Here's how the part is built. I have some questions about the finished solid (model axes, mm). Face numbers are marked on the shaded views. A direction names the side the tool comes from. Coordinates: 2 decimals unless noted, no trailing zeros. Order: outer loops, then holes, each group sorted by start corner. A loop starts at its lowest first (then second) coordinate and runs counter-clockwise, first axis right, second up. Notation, with made-up numbers: (-28.75, 24) -> (8.25, 24) arc R16 ccw to (8.25, 53) -> close; hole circle Ø5 at (81.25, 15). An arc over 180 degrees is marked (long way). One line per item, written item: value. Start each with the question number.
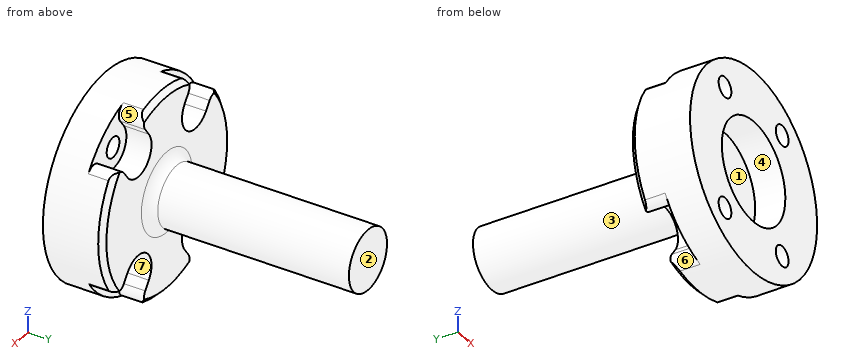
```python
from build123d import *

# Parameters (mm, degrees)
SKETCH_2_R          = 1.0000000000000002
SKETCH_2_R_2        = 0.9999999999999998
CUT_EXTRUDE_1_DEPTH = 10
SKETCH_3_R          = 1.0000000000000002
SKETCH_3_R_2        = 0.9999999999999998
CUT_EXTRUDE_2_DEPTH = 2.5
FILLET_1_R          = 1
FILLET_2_R          = 1


with BuildPart() as part:
    # 草图1 → 旋转1 (revolve)
    with BuildSketch(Plane.XY, mode=Mode.PRIVATE) as revolve_1_sk:
        Polygon((-1.97e-15, 26), (2.999999999999997, 26), (3, 6), (9.5, 5.999999999999999), (10.000000000000002, 5.5), (10, -1.2e-16), (5.000000000000001, -6.1e-16), (5.000000000000002, 2.9999999999999996), (8.7e-16, 2.999999999999999), align=None)
    revolve(revolve_1_sk.sketch.rotate(Axis((0, 9.947317903416637, 0), (0, -1, 0)), 90), axis=Axis((0, 9.947317903416637, 0), (0, -1, 0)))

    # 草图2 → 切除-拉伸1 (cut)
    with BuildSketch(Plane(origin=(0, 6, 0), x_dir=(1, 0, 0), z_dir=(0, 1, 0))):
        with Locations(Location((-4.5, 6.000000000000001, 0), (0, 0, 270))):
            Circle(SKETCH_2_R)
        with Locations(Location((4.5, 6.000000000000003, 0), (0, 0, 270))):
            Circle(SKETCH_2_R_2)
        with Locations(Location((4.5, -5.999999999999997, 0), (0, 0, 270))):
            Circle(SKETCH_2_R_2)
        with Locations(Location((-4.5, -5.999999999999999, 0), (0, 0, 270))):
            Circle(SKETCH_2_R)
    extrude(amount=-CUT_EXTRUDE_1_DEPTH, mode=Mode.SUBTRACT)

    # 草图3 → 切除-拉伸2 (cut)
    # profile 1 of 8: a face of its own
    with BuildSketch(Plane(origin=(0, 6, 0), x_dir=(1, 0, 0), z_dir=(0, 1, 0))):
        with BuildLine():
            Line((-9.157565431651806, 8.710087242202405), (-7.2389927145122455, 6.151990286016327))
            ThreePointArc((-7.2389927145121735, 6.151990286016362), (-5.700000000000015, 7.599999999999989), (-3.8789927145123357, 8.67199028601625))
            Line((-3.8789927145122554, 8.67199028601634), (-5.797565431651803, 11.230087242202407))
            Line((-5.797565431651803, 11.230087242202407), (-9.157565431651806, 8.710087242202405))
        make_face()
    # profile 2 of 8: a face of its own
    with BuildSketch(Plane(origin=(0, 6, 0), x_dir=(1, 0, 0), z_dir=(0, 1, 0))):
        with BuildLine():
            ThreePointArc((-3.8789927145123357, 8.67199028601625), (-5.700000000000015, 7.599999999999989), (-7.2389927145121735, 6.151990286016362))
            Line((-7.2389927145122455, 6.151990286016327), (-6.18, 4.739999999999999))
            ThreePointArc((-6.18, 4.739999999999998), (-3.24, 4.3199999999999985), (-2.819999999999999, 7.259999999999998))
            Line((-2.819999999999999, 7.259999999999998), (-3.8789927145122554, 8.67199028601634))
        make_face()
        with Locations(Location((-4.5, 6.000000000000001, 0), (0, 0, 270))):
            Circle(SKETCH_3_R, mode=Mode.SUBTRACT)
    # profile 3 of 8: a face of its own
    with BuildSketch(Plane(origin=(0, 6, 0), x_dir=(1, 0, 0), z_dir=(0, 1, 0))):
        with BuildLine():
            ThreePointArc((7.2389927145121815, 6.1519902860163524), (5.700000000000022, 7.599999999999984), (3.878992714512337, 8.67199028601625))
            Line((3.8789927145122567, 8.671990286016342), (2.819999999999999, 7.259999999999998))
            ThreePointArc((2.8199999999999985, 7.259999999999998), (3.24, 4.319999999999999), (6.18, 4.739999999999999))
            Line((6.18, 4.739999999999999), (7.238992714512243, 6.151990286016323))
        make_face()
        with Locations(Location((4.5, 6.000000000000003, 0), (0, 0, 270))):
            Circle(SKETCH_3_R_2, mode=Mode.SUBTRACT)
    # profile 4 of 8: a face of its own
    with BuildSketch(Plane(origin=(0, 6, 0), x_dir=(1, 0, 0), z_dir=(0, 1, 0))):
        with BuildLine():
            Line((5.797565431651803, 11.230087242202407), (3.8789927145122567, 8.671990286016342))
            ThreePointArc((3.878992714512337, 8.67199028601625), (5.700000000000022, 7.599999999999984), (7.2389927145121815, 6.1519902860163524))
            Line((7.238992714512243, 6.151990286016323), (9.157565431651806, 8.710087242202405))
            Line((9.157565431651806, 8.710087242202405), (5.797565431651803, 11.230087242202407))
        make_face()
    # profile 5 of 8: a face of its own
    with BuildSketch(Plane(origin=(0, 6, 0), x_dir=(1, 0, 0), z_dir=(0, 1, 0))):
        with BuildLine():
            Line((2.819999999999999, -7.259999999999998), (3.8789927145122527, -8.671990286016337))
            ThreePointArc((3.8789927145123175, -8.671990286016259), (5.700000000000012, -7.599999999999992), (7.238992714512178, -6.151990286016356))
            Line((7.238992714512243, -6.151990286016323), (6.18, -4.739999999999999))
            ThreePointArc((6.18, -4.739999999999999), (3.24, -4.319999999999999), (2.8199999999999985, -7.259999999999998))
        make_face()
        with Locations(Location((4.5, -5.999999999999997, 0), (0, 0, 270))):
            Circle(SKETCH_3_R_2, mode=Mode.SUBTRACT)
    # profile 6 of 8: a face of its own
    with BuildSketch(Plane(origin=(0, 6, 0), x_dir=(1, 0, 0), z_dir=(0, 1, 0))):
        with BuildLine():
            ThreePointArc((7.238992714512178, -6.151990286016356), (5.700000000000012, -7.599999999999992), (3.8789927145123175, -8.671990286016259))
            Line((3.8789927145122527, -8.671990286016337), (5.797565431651803, -11.230087242202407))
            Line((5.797565431651803, -11.230087242202407), (9.157565431651806, -8.710087242202405))
            Line((9.157565431651806, -8.710087242202405), (7.238992714512243, -6.151990286016323))
        make_face()
    # profile 7 of 8: a face of its own
    with BuildSketch(Plane(origin=(0, 6, 0), x_dir=(1, 0, 0), z_dir=(0, 1, 0))):
        with BuildLine():
            ThreePointArc((-2.819999999999999, -7.259999999999998), (-2.4211060633115498, -5.703015151901651), (-3.239999999999995, -4.320000000000003))
            ThreePointArc((-3.239999999999995, -4.320000000000003), (-4.796984848098346, -3.921106063311549), (-6.18, -4.739999999999998))
            Line((-6.18, -4.739999999999999), (-7.238992714512246, -6.151990286016328))
            ThreePointArc((-7.238992714512174, -6.15199028601636), (-5.7000000000000135, -7.59999999999999), (-3.8789927145123286, -8.671990286016255))
            Line((-3.8789927145122527, -8.671990286016337), (-2.819999999999999, -7.259999999999998))
        make_face()
        with BuildLine():
            ThreePointArc((-3.5, -5.999999999999999), (-5.3944271909999175, -6.447213595499955), (-3.899999999999996, -5.200000000000002))
            ThreePointArc((-3.899999999999996, -5.200000000000002), (-3.605572809000083, -5.5527864045000435), (-3.5, -5.999999999999999))
        make_face(mode=Mode.SUBTRACT)
    # profile 8 of 8: a face of its own
    with BuildSketch(Plane(origin=(0, 6, 0), x_dir=(1, 0, 0), z_dir=(0, 1, 0))):
        with BuildLine():
            ThreePointArc((-3.8789927145123286, -8.671990286016255), (-5.7000000000000135, -7.59999999999999), (-7.238992714512174, -6.15199028601636))
            Line((-7.238992714512246, -6.151990286016328), (-9.157565431651806, -8.710087242202405))
            Line((-9.157565431651806, -8.710087242202405), (-5.797565431651803, -11.230087242202407))
            Line((-5.797565431651803, -11.230087242202407), (-3.8789927145122527, -8.671990286016337))
        make_face()
    extrude(amount=-CUT_EXTRUDE_2_DEPTH, mode=Mode.SUBTRACT)

    # 圆角1
    fillet_1_edges = [part.edges().sort_by_distance(p)[0] for p in [
        (7.5462083154282915, 4.5, -6.56161108723772),
        (4.18620831542829, 4.5, -9.08161108723772),
        (4.18620831542829, 4.5, 9.08161108723772),
        (7.5462083154282915, 4.5, 6.561611087237719),
        (-4.18620831542829, 4.5, 9.08161108723772),
        (-7.546208315428291, 4.5, 6.56161108723772),
        (-7.54620831542829, 4.5, -6.561611087237719),
        (-4.186208315428289, 4.5, -9.08161108723772),
    ]]
    fillet(fillet_1_edges, radius=FILLET_1_R)

    # 圆角2
    fillet_2_edges = [part.edges().sort_by_distance(p)[0] for p in [
        (-7e-16, 6, -3),
    ]]
    fillet(fillet_2_edges, radius=FILLET_2_R)


solid = part.part
```
Q1. Imagine slicing it at B-B (x = 4.5). Write out the boundary of the cut face in (y, z).
Q2. Imagine slicing it at A-A (z = -6.5). Write out the boundary of the cut face in (x, y), plus the area to 3 significant figures.
Q3. Imagine slicing it at D-D (x = 0). Write out the boundary of the cut face in (y, z).
Q4. For P1, Ø5, axis at x = 6.5, z = -5.5, coming from the +Y side; P2, Ø4, axis at x = -2, y = 7, coming from the +Z side; P3, Ø6, axis at x = -3.5, y = 12.5, coming from the -Z side, each with a flat end and sliding along its axis, tell me the tip position at first contact or that it passes through.
Q5. I need wall thicknesses on line 1 (X direction, y = 2.1, z = 0); line 2 (X direction, y = 2.25, z = 6); line 3 (Y direction, x = 7.5, z = -3.5). Which ranges of each line are inside material? Lowest first, please.
Q6. Imagine slicing it at C-C (z = 0). Write out the boundary of the cut face in (x, y), plus the area to 3 significant figures.
Q7. For the marked faces 4, 5, 6 and 7, which set-ups out of +Z, -Z, +X, -X, +Y, -Y let a thin tool reach every point of the face, with its end or its side?
Q8. If we mould it in two halves opening along Z, with no side actions, what happens to the marked faces 1, 2 and 3? For each: +Z half, -Z half, draft (parallel to the pull), parting line (faces both ways), or undercut.
Completed:
1. outline: (0, -8.93) -> (3.5, -8.93) -> (3.5, -7) -> (0, -7) -> close; (0, -5) -> (3.5, -5) -> (3.5, -3.9) -> (6, -3.9) -> (6, 3.9) -> (3.5, 3.9) -> (3.5, 5) -> (0, 5) -> (0, 2.18) -> (3, 2.18) -> (3, -2.18) -> (0, -2.18) -> close; (0, 7) -> (3.5, 7) -> (3.5, 8.93) -> (0, 8.93) -> close
2. outline: (-7.6, 0) -> (-5.37, 0) -> (-5.37, 3.5) -> (-7.6, 3.5) -> close; (-3.63, 0) -> (3.63, 0) -> (3.63, 3.5) -> (2.46, 3.5) -> (2.46, 6) -> (-2.46, 6) -> (-2.46, 3.5) -> (-3.63, 3.5) -> close; (5.37, 0) -> (7.6, 0) -> (7.6, 3.5) -> (5.37, 3.5) -> close
2. area: 53.4 mm2
3. outline: (0, -10) -> (5.5, -10) -> (6, -9.5) -> (6, -4) arc R1 cw to (7, -3) -> (26, -3) -> (26, 3) -> (7, 3) arc R1 cw to (6, 4) -> (6, 9.5) -> (5.5, 10) -> (0, 10) -> (0, 5) -> (3, 5) -> (3, -5) -> (0, -5) -> close
4. P1: stops at y = 6
4. P2: stops at z = 9.98
4. P3: stops at z = -2.96
5. line 1: x = -10 to -5, 5 to 10
5. line 2: x = -8 to -5.5, -3.5 to 3.5, 5.5 to 8
5. line 3: y = 0 to 6
6. outline: (-10, 0) -> (-5, 0) -> (-5, 3) -> (5, 3) -> (5, 0) -> (10, 0) -> (10, 5.5) -> (9.5, 6) -> (4, 6) arc R1 cw to (3, 7) -> (3, 26) -> (-3, 26) -> (-3, 7) arc R1 cw to (-4, 6) -> (-9.5, 6) -> (-10, 5.5) -> close
6. area: 210 mm2
7. face 4: -Y
7. face 5: +X, +Y
7. face 6: -X, +Y
7. face 7: +Y
8. face 1: undercut
8. face 2: draft
8. face 3: parting line
